Geometry: final body of the model. Coordinates: model frame, mm. Give positions to 0.01 mm unless a question says otherwise; leave off trailing zeros. Write each loop counter-clockwise with the first axis right and the second up, starting at its lowest first coordinate (ties: lowest second). Pieces come first, ordered by that corner, then holes.
```python
from build123d import *

# Parameters (mm, degrees)
F1_DEPTH = 1.016
F2_DEPTH = 17.78
F3_R     = 2.0447
F3_R_2   = 2.0406784107
F4_DEPTH = 12.7


# Not quite as in the source:
# - a feature names something its author has since deleted; it is built from what else it names


with BuildPart() as f1:
    # F0 (on Front) → F1 (new body)
    with BuildSketch(Plane.XZ):
        Polygon((-27.083877352, 12.2783370181), (26.9169844677, 12.2783370181), (0, 55.663280189), align=None)
    extrude(amount=F1_DEPTH)

    # F2 (add): a face of the model
    f2_faces = [f1.faces().sort_by_distance(p)[0] for p in [
        (-0.0556309614, -1.016, 26.7399847417),
    ]]
    extrude(f2_faces, amount=F2_DEPTH)

    # F3 (on face) → F4 (cut)
    with BuildSketch(Plane.XZ.offset(18.796)):
        with Locations((3.6953620147, 41.2761941552)):
            Circle(F3_R)
        with Locations((0, 48.6748889089)):
            Circle(F3_R_2)
        with Locations((-4.3132207356, 41.2761941552)):
            Circle(F3_R)
        with Locations((0, 33.7593667209)):
            Circle(F3_R)
        with Locations((7.9806558788, 33.7593667209)):
            Circle(F3_R)
        with Locations((-8.3175115287, 33.7593667209)):
            Circle(F3_R)
        with Locations((-4.3132207356, 25.8912853897)):
            Circle(F3_R)
        with Locations((-14.0078207478, 25.8912853897)):
            Circle(F3_R)
        with Locations((3.8358634338, 25.8912853897)):
            Circle(F3_R)
        with Locations((11.9849471375, 25.8912853897)):
            Circle(F3_R)
        with Locations((18.096761778, 17.2504447401)):
            Circle(F3_R)
        with Locations((8.6129121482, 17.2504447401)):
            Circle(F3_R)
        with Locations((0, 17.2504447401)):
            Circle(F3_R)
        with Locations((-8.3175115287, 17.2504447401)):
            Circle(F3_R)
        with Locations((-18.1526131928, 17.2504447401)):
            Circle(F3_R)
    extrude(amount=-F4_DEPTH, mode=Mode.SUBTRACT)


solid = f1.part
```
Item 1: Section B-B, the plane x = 17. Return the cut outline in (y, z), plus the area to 3 significant figures.
Found:
outline: (-18.8, 12.28) - (0, 12.28) - (0, 28.26) - (-18.8, 28.26) - (-18.8, 18.98) - (-6.1, 18.98) - (-6.1, 15.52) - (-18.8, 15.52) - close
area: 257 mm2
Item 2: Section D-D, the plane z = 31. Return the cut outline in (x, y), plus the area to 3 significant figures.
Found:
outline: (-15.4, -18.8) - (15.3, -18.8) - (15.3, 0) - (-15.4, 0) - close
area: 577 mm2
Item 3: Pull-direction query (X, two-part tool) for faces 1 (the face through (13.647, -9.266, 33.667)), 2 (the face through (0, 0, 29)), 3 (the face through (0, -6.096, 17)); classes: +X half, -X half, draft (parallel to the pull), parting line (faces both ways), or undercut.
Found:
face 1: +X half
face 2: draft
face 3: undercut
Item 4: Pin query (flat end, axial travel): pin 1 Ø4 at (x, z) = (3.5, 17) entering from +Y; pin 2 Ø5 at (y, z) = (-3, 23.5) entering from +X; pin 3 Ø1.2 at (x, z) = (-19, 17) entering from -Y; pin 4 Ø1.5 at (y, z) = (-13.5, 41.5) entering from -X. Return the tip coordinate at first contact, or that it passes through.
Found:
pin 1: stops at y = 0
pin 2: stops at x = 21.51
pin 3: stops at y = -6.1
pin 4: stops at x = -9.31
Item 5: Line query: L1, parallel to X at y = -17.5, z = 32.5; L2, parallel to X at y = -8.5, z = 18; L3, parallel to X at y = -7, z = 16.5. Output: solid intervals per line, ascending.
Found:
L1: x = -14.46 to -9.93, -6.71 to -1.61, 1.61 to 6.37, 9.59 to 14.37
L2: x = -23.51 to -20.05, -16.25 to -10.22, -6.42 to -1.9, 1.9 to 6.71, 10.52 to 16.19, 20 to 23.37
L3: x = -24.45 to -20.05, -16.25 to -10.22, -6.42 to -1.9, 1.9 to 6.71, 10.51 to 16.19, 20 to 24.3
Item 6: Section A-A, the plane y = -13. State how many separate pieces and enclosed holes the cut face has, plus the area to 3 significant figures.
Found:
separate pieces: 1
enclosed holes: 15
area: 974 mm2
Item 7: Section C-C, the plane y = -2.5. Return the cut outline in (x, z).
Found:
outline: (-27.08, 12.28) - (26.92, 12.28) - (0, 55.66) - close
